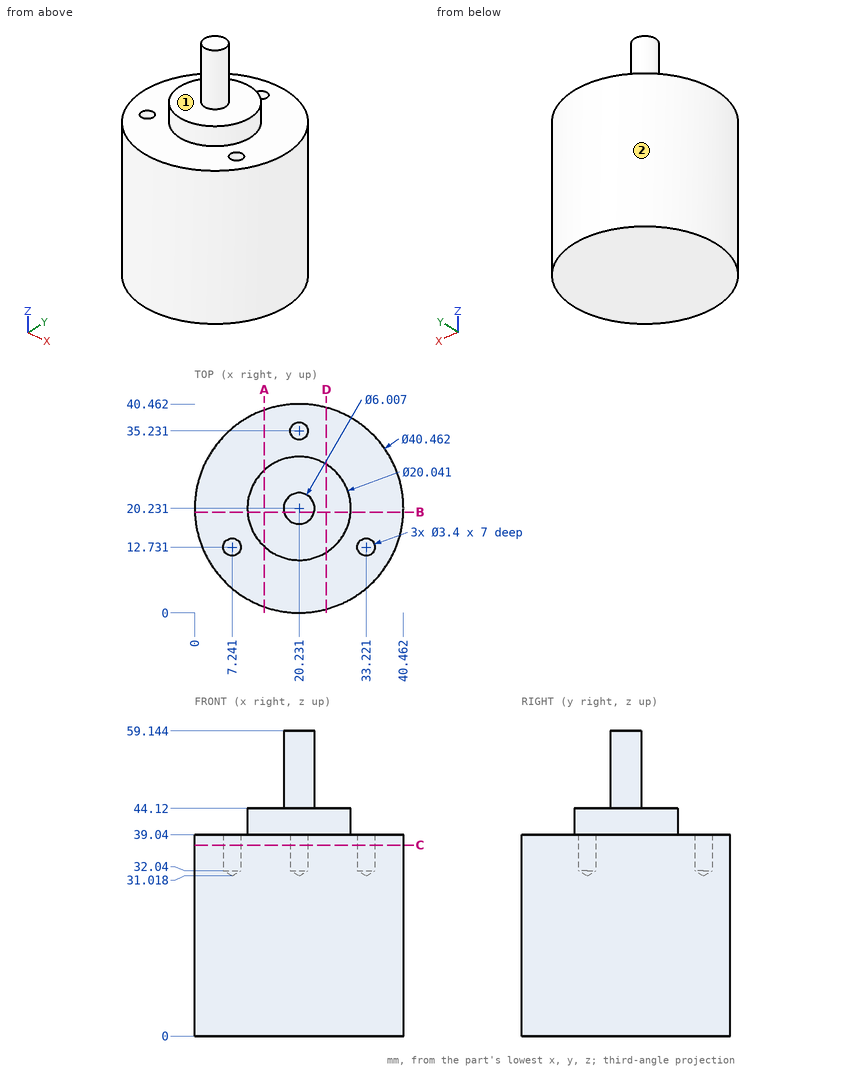
Geometry check sheet. Reference: drawing and pictorial views, mm from the part's lowest x, y, z. A direction names the side the tool comes from. Round coordinates to 2 decimals unless told otherwise and drop trailing zeros. Loops run counter-clockwise (first coordinate to the right, second up) from the corner with the lowest first, then second, coordinate; pieces in that order, holes last.
1. Set-up check for the marked faces 1 and 2: record each of +Z, -Z, +X, -X, +Y, -Y from which the full face is reachable in a straight line by a thin tool's end or side.
2. Sectioned sample at D-D on x = 25.5. Record the boundary of the cut face in (y, z) (1 decimal), and give its area (3 significant figures).
3. Gauge pin test, flat ends, axial feed: pin 1 Ø5.5 at (x, y) = (20.23, 35.23) entering from +Z; pin 2 Ø1 at (x, z) = (25, 37) entering from +Y; pin 3 Ø1.5 at (x, y) = (19.5, 14.5) entering from -Z; pin 4 Ø4 at (y, z) = (15.5, 49) entering from -X. Record the tip position at first contact, or that the pin passes through.
4. Sectioned sample at B-B on y = 19.5. Record the boundary of the cut face in (x, z) (1 decimal), and give its area (3 significant figures).
5. Scan lines: probe 1 along Z at (x, y) = (14.5, 10); probe 2 along Z at (x, y) = (27, 27); probe 3 along Y at (x, z) = (20, 51) (1 decimal). Record each from-to range of solid material in increasing order.
6. Sectioned sample at A-A on x = 13.5. Record the boundary of the cut face in (y, z).
7. Sectioned sample at C-C on z = 37. Record the boundary of the cut face in (x, y), and give its area (3 significant figures).
Recorded:
1. face 1: +Z
1. face 2: +Z, -Z
2. outline: (0.7, 0) - (39.8, 0) - (39.8, 39) - (28.8, 39) - (28.8, 44.1) - (11.7, 44.1) - (11.7, 39) - (0.7, 39) - close
2. area: 1,610 mm2
3. pin 1: stops at z = 39.04
3. pin 2: stops at y = 40.01
3. pin 3: stops at z = 0
3. pin 4: stops at x = 18.98
4. outline: (0, 0) - (40.4, 0) - (40.4, 39) - (30.2, 39) - (30.2, 44.1) - (23.1, 44.1) - (23.1, 59.1) - (17.3, 59.1) - (17.3, 44.1) - (10.2, 44.1) - (10.2, 39) - (0, 39) - close
4. area: 1,770 mm2
5. probe 1: z = 0 to 39.04
5. probe 2: z = 0 to 44.12
5. probe 3: y = 17.2 to 23.2
6. outline: (1.15, 0) - (39.31, 0) - (39.31, 39.04) - (27.65, 39.04) - (27.65, 44.12) - (12.81, 44.12) - (12.81, 39.04) - (1.15, 39.04) - close
7. outline: circle Ø40.46 at (20.23, 20.23); hole circle Ø3.4 at (7.24, 12.73); hole circle Ø3.4 at (20.23, 35.23); hole circle Ø3.4 at (33.22, 12.73)
7. area: 1,260 mm2
